```python
from build123d import *

# Parameters (mm, degrees)
F0_W      = 35.5
F0_H      = 25.5
F1_DEPTH  = 25.5
F2_W      = 20.5
F2_H      = 20.5
F3_DEPTH  = 35.5
F4_W      = 15.5
F4_H      = 25.5
F5_DEPTH  = 25
F6_W      = 20.5
F6_H      = 20.5
F7_DEPTH  = 38
F8_R      = 2.65
F9_DEPTH  = 2
F10_R     = 1.65
F11_DEPTH = 27.501
F12_R     = 2.7
F13_DEPTH = 2
F14_R     = 1.65
F15_DEPTH = 5.5
F16_W     = 2.5
F16_H     = 25
F17_DEPTH = 20.5
F18_W     = 20
F18_H     = 20.5
F19_DEPTH = 2.5
F20_W     = 2.5
F20_H     = 2.5
F21_DEPTH = 20.5
F22_W     = 7.5
F22_H     = 20.5
F23_DEPTH = 2.5
F24_W     = 10
F24_H     = 20.5
F25_DEPTH = 2.5
F26_W     = 10
F26_H     = 20.5
F27_DEPTH = 2.5
F28_W     = 9
F28_H     = 20.5
F28_W_2   = 8.5
F29_DEPTH = 2.5


with BuildPart() as f1:
    # F0 (on Front) → F1 (new body)
    with BuildSketch(Plane.XZ):
        Rectangle(F0_W, F0_H)
    extrude(amount=F1_DEPTH)

    # F2 (on face) → F3 (cut)
    with BuildSketch(Plane(origin=(-17.75, 0, 0), x_dir=(0, -1, 0), z_dir=(-1, 0, 0))):
        with Locations((12.75, 0)):
            Rectangle(F2_W, F2_H)
    extrude(amount=-F3_DEPTH, mode=Mode.SUBTRACT)

    # F4 (on face) → F5 (join)
    with BuildSketch(Plane.XZ.offset(25.5)):
        Rectangle(F4_W, F4_H)
    extrude(amount=F5_DEPTH)

    # F6 (on face) → F7 (cut)
    with BuildSketch(Plane.XZ.offset(50.5)):
        with Locations((-5, 0)):
            Rectangle(F6_W, F6_H)
    extrude(amount=-F7_DEPTH, mode=Mode.SUBTRACT)

    # F8 (on face) → F9 (join)
    with BuildSketch(Plane.YZ.offset(7.75)):
        with Locations((-38, 0)):
            Circle(F8_R)
    extrude(amount=F9_DEPTH)

    # F10 (on face) → F11 (cut, through all)
    with BuildSketch(Plane.YZ.offset(9.75)):
        with Locations((-38, 0)):
            Circle(F10_R)
    extrude(amount=-F11_DEPTH, mode=Mode.SUBTRACT)

    # F12 (on face) → F13 (join)
    with BuildSketch(Plane(origin=(0, 0, 0), x_dir=(-1, 0, 0), z_dir=(0, 1, 0))):
        Circle(F12_R)
    extrude(amount=F13_DEPTH)

    # F14 (on face) → F15 (cut)
    with BuildSketch(Plane(origin=(0, 2, 0), x_dir=(-1, 0, 0), z_dir=(0, 1, 0))):
        Circle(F14_R)
    extrude(amount=-F15_DEPTH, mode=Mode.SUBTRACT)

    # F16 (on face) → F17 (join)
    with BuildSketch(Plane.XY.offset(-10.25)):
        with Locations((-6.5, -38)):
            Rectangle(F16_W, F16_H)
    extrude(amount=F17_DEPTH)

    # F18 (on face) → F19 (cut)
    with BuildSketch(Plane(origin=(-7.75, 0, 0), x_dir=(0, -1, 0), z_dir=(-1, 0, 0))):
        with Locations((38, 0)):
            Rectangle(F18_W, F18_H)
    extrude(amount=-F19_DEPTH, mode=Mode.SUBTRACT)

    # F20 (on face) → F21 (join)
    with BuildSketch(Plane.XY.offset(-10.25)):
        with Locations((-6.5, -38.25)):
            Rectangle(F20_W, F20_H)
    extrude(amount=F21_DEPTH)

    # F22 (on face) → F23 (cut)
    with BuildSketch(Plane.XZ.offset(25.5)):
        with Locations((11.5, 0)):
            Rectangle(F22_W, F22_H)
    extrude(amount=-F23_DEPTH, mode=Mode.SUBTRACT)

    # F24 (on face) → F25 (join)
    with BuildSketch(Plane.XZ.offset(25.5)):
        with Locations((-10.25, 0)):
            Rectangle(F24_W, F24_H)
    extrude(amount=-F25_DEPTH)

    # F26 (on face) → F27 (join)
    with BuildSketch(Plane.XZ.offset(25.5)):
        with Locations((10.25, 0)):
            Rectangle(F26_W, F26_H)
    extrude(amount=-F27_DEPTH)

    # F28 (on face) → F29 (join)
    with BuildSketch(Plane(origin=(-7.75, 0, 0), x_dir=(0, -1, 0), z_dir=(-1, 0, 0))):
        with Locations((32.5, 0)):
            Rectangle(F28_W, F28_H)
        with Locations((43.75, 0)):
            Rectangle(F28_W_2, F28_H)
    extrude(amount=-F29_DEPTH)


solid = f1.part
```
Geometry check sheet. Reference: the model listing, model coordinates, mm. A direction names the side the tool comes from. Round coordinates to 2 decimals unless told otherwise and drop trailing zeros. Loops run counter-clockwise (first coordinate to the right, second up) from the corner with the lowest first, then second, coordinate; pieces in that order, holes last. Notation, with made-up numbers: (15, 81.25) -> (60, 81.25) arc R20 ccw to (60, 109.25) -> close; hole circle Ø1 at (47.25, 82). An arc over 180 degrees is marked (long way). Use a Markdown table: item, result.
(1) Go/stop test with flat-tipped pins: P1, Ø13, axis at x = 8.5, z = 5, coming from the +Y side; P2, Ø4, axis at y = -37, z = 0.5, coming from the +X side; P3, Ø2.5, axis at y = -38, z = 0, coming from the -X side. Record where each tip stops, or that it passes through.
Calculated:
| item | result |
|---|---|
| P1 | y = 0 |
| P2 | x = 9.75 |
| P3 | x = -7.75 |
(2) Scan lines: probe 1 along Z at (x, y) = (5, -34.5); probe 2 along Y at (x, z) = (9.5, -7.5); probe 3 along Z at (x, y) = (0, -1.6). Record each from-to range of solid material in increasing order.
Calculated:
| item | result |
|---|---|
| probe 1 | -12.75 to -10.25, 10.25 to 12.75 |
| probe 2 | -25.5 to -23, -2.5 to 0 |
| probe 3 | -12.75 to -1.65, 1.65 to 12.75 |
(3) Set-up check for faces 1 (the flat face through (-5.25, -37, 0)), 2 (the cylindrical face through (8.736, -40.647, 0.117)), 3 (the flat face through (9.75, -38, -2)), 4 (the flat face through (11, -23, 0)), 5 (the cylindrical face through (0.585, 0.986, -2.636)): record each of +Z, -Z, +X, -X, +Y, -Y from which the full face is reachable in a straight line by a thin tool's end or side.
Calculated:
| item | result |
|---|---|
| face 1 | -Y |
| face 2 | +X |
| face 3 | +Z, -Z, +X, -Y |
| face 4 | +X, -X |
| face 5 | +Y |
(4) Sectioned sample at A-A (z = -8.25). Enter the section's corners in (x, y), then the cut area to 3 significant figures.
Calculated:
| item | result |
|---|---|
| outline | (-17.75, -25.5) -> (-7.75, -25.5) -> (-7.75, -50.5) -> (-5.25, -50.5) -> (-5.25, -23) -> (-17.75, -23) -> close; (-17.75, -2.5) -> (17.75, -2.5) -> (17.75, 0) -> (-17.75, 0) -> close; (5.25, -50.5) -> (7.75, -50.5) -> (7.75, -25.5) -> (17.75, -25.5) -> (17.75, -23) -> (5.25, -23) -> close |
| area | 276 mm² |
(5) Sectioned sample at B-B (y = -13). Enter the section's corners in (x, z), then the cut area to 4 significant figures.
Calculated:
| item | result |
|---|---|
| outline | (-17.75, -12.75) -> (17.75, -12.75) -> (17.75, -10.25) -> (-17.75, -10.25) -> close; (-17.75, 10.25) -> (17.75, 10.25) -> (17.75, 12.75) -> (-17.75, 12.75) -> close |
| area | 177.5 mm² |
(6) Sectioned sample at D-D (z = 0). Give the number of separate pieces and of enclosed holes in the cut face, then the cut area to 3 significant figures.
Calculated:
| item | result |
|---|---|
| separate pieces | 5 |
| enclosed holes | 0 |
| area | 268 mm² |
(7) Mould release check, pull along Y, two halves, no side actions. Record for faces 6 (the flat face through (0, -21, -10.25)), 7 (the flat face through (0, 0, 3)), 8 (the flat face through (-13, -25.5, 0)): released by +Y, released by -Y, zero draft, split by the parting line, or undercut.
Calculated:
| item | result |
|---|---|
| face 6 | undercut |
| face 7 | released by +Y |
| face 8 | released by -Y |
(8) Sectioned sample at C-C (x = 12). Enter the section's corners in (y, z).
Calculated:
| item | result |
|---|---|
| outline | (-25.5, -12.75) -> (0, -12.75) -> (0, 12.75) -> (-25.5, 12.75) -> close; hole (-23, -10.25) -> (-2.5, -10.25) -> (-2.5, 10.25) -> (-23, 10.25) -> close |
